```python
from build123d import *

# Parameters (mm, degrees)
SKETCH_1_W                  = 310
SKETCH_1_H                  = 40
EXTRUDE_1_DEPTH             = 12
SKETCH_8_W                  = 95
SKETCH_8_H                  = 15
SKETCH_8_W_2                = 310
EXTRUDE_2_DEPTH             = 12
HOLE_WIZARD_2_D             = 9
HOLE_WIZARD_2_CBORE_D       = 14
HOLE_WIZARD_2_CBORE_DEPTH   = 9
HOLE_WIZARD_2_2_D           = 9
HOLE_WIZARD_2_2_CBORE_D     = 14
HOLE_WIZARD_2_2_CBORE_DEPTH = 9
HOLE_WIZARD_3_D             = 6.5
HOLE_WIZARD_3_CBORE_D       = 11
HOLE_WIZARD_3_CBORE_DEPTH   = 7
CUT_EXTRUDE_1_DEPTH         = 13


with BuildPart() as part:
    # 草图1 → 凸台-拉伸1 (new body)
    with BuildSketch(Plane.XY):
        Rectangle(SKETCH_1_W, SKETCH_1_H)
    extrude(amount=EXTRUDE_1_DEPTH)

    # 草图8 → 凸台-拉伸2 (add)
    with BuildSketch(Plane.XY.offset(12)):
        with Locations((-107.5, 27.5)):
            Rectangle(SKETCH_8_W, SKETCH_8_H)
        with Locations((107.5, 27.5)):
            Rectangle(SKETCH_8_W, SKETCH_8_H)
        with Locations((0, -27.5)):
            Rectangle(SKETCH_8_W_2, SKETCH_8_H)
    extrude(amount=-EXTRUDE_2_DEPTH)

    # Hole Wizard 2 (through all)
    with Locations(Plane.XY.offset(12)):
        with Locations((-126, 22.5), (-69, 22.5), (-69, -22.5), (-126, -22.5), (126, -22.5), (69, -22.5), (69, 22.5), (126, 22.5)):
            CounterBoreHole(HOLE_WIZARD_2_D / 2, HOLE_WIZARD_2_CBORE_D / 2, HOLE_WIZARD_2_CBORE_DEPTH)

    # Hole Wizard 2 2 (through all)
    with Locations(Plane(origin=(0, 0, 0), x_dir=(-1, 0, 0), z_dir=(0, 0, -1))):
        with Locations((-142.5, 15), (-142.5, -15), (142.5, -15), (142.5, 15)):
            CounterBoreHole(HOLE_WIZARD_2_2_D / 2, HOLE_WIZARD_2_2_CBORE_D / 2, HOLE_WIZARD_2_2_CBORE_DEPTH)

    # 打孔尺寸(%根据)内六角圆柱头螺钉的类型3 (through all)
    with Locations(Plane(origin=(0, 0, 0), x_dir=(-1, 0, 0), z_dir=(0, 0, -1))):
        with Locations((-82, 27.5), (-113, 27.5), (-113, -27.5), (-82, -27.5), (82, -27.5), (113, -27.5), (113, 27.5), (82, 27.5)):
            CounterBoreHole(HOLE_WIZARD_3_D / 2, HOLE_WIZARD_3_CBORE_D / 2, HOLE_WIZARD_3_CBORE_DEPTH)

    # 草图11 → 切除-拉伸1 (cut, through all)
    with BuildSketch(Plane.XY.offset(12)):
        with BuildLine():
            Line((-60, 20), (60, 20))
            Line((60, 20), (60, 0))
            ThreePointArc((60, 0), (58.535533906, -3.535533906), (55, -5))
            Line((55, -5), (-55, -5))
            ThreePointArc((-55, -5), (-58.535533906, -3.535533906), (-60, 0))
            Line((-60, 0), (-60, 20))
        make_face()
    extrude(amount=-CUT_EXTRUDE_1_DEPTH, mode=Mode.SUBTRACT)


solid = part.part
```
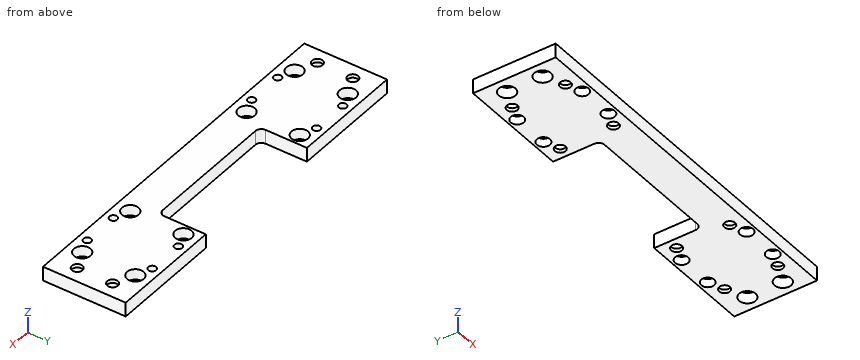
Check sheet for the modelled part. Datum: model origin and axes. Units: mm. Round coordinates to 2 decimals unless told otherwise and drop trailing zeros. Loops run counter-clockwise (first coordinate to the right, second up) from the corner with the lowest first, then second, coordinate; pieces in that order, holes last. Notation, with made-up numbers: M 76.25,-6 L 127.25,-6 A8 ccw 127.25,5 Z; hole C -2.5,87 d2. An arc over 180 degrees is marked long. Answer as a JSON object with one key per item and string values.
1. Section check B-B (z = 5). State how many separate pieces and enclosed holes the cut face has, plus the area to 3 significant figures.
Reply:
{"separate pieces": "1", "enclosed holes": "20", "area": "14,300 mm²"}
2. Scan lines: line 1 (Y direction, x = -82, z = 3); line 2 (Y direction, x = 69, z = 0.8); line 3 (X direction, y = -9.5, z = 5). Record each from-to range of solid material in increasing order.
Reply:
{"line 1": "y = -35 to -33, -22 to 22, 33 to 35", "line 2": "y = -35 to -27, -18 to 18, 27 to 35", "line 3": "x = -155 to -146.83, -138.17 to 138.17, 146.83 to 155"}
3. Section check A-A (x = -82). Record the boundary of the cut face in (y, z).
Reply:
{"outline": "M -35,0 L -33,0 L -33,7 L -30.75,7 L -30.75,12 L -35,12 Z; M -24.25,7 L -22,7 L -22,0 L 22,0 L 22,7 L 24.25,7 L 24.25,12 L -24.25,12 Z; M 30.75,7 L 33,7 L 33,0 L 35,0 L 35,12 L 30.75,12 Z"}
4. Gauge pin test, flat ends, axial feed: P1, Ø10.5, axis at x = 82, y = 27.5, coming from the -Z side; P2, Ø22.5, axis at x = 69, y = 22.5, coming from the +Z side; P3, Ø4, axis at x = 45.5, z = 3, coming from the +Y side. Record the tip position at first contact, or that the pin passes through.
Reply:
{"P1": "stops at z = 7", "P2": "stops at z = 12", "P3": "stops at y = -5"}
